Check sheet for the drawn part. Datum: minimum x, y, z corner. Units: mm. Round coordinates to 2 decimals unless told otherwise and drop trailing zeros. Write each loop counter-clockwise with the first axis right and the second up, starting at its lowest first coordinate (ties: lowest second). Pieces come first, ordered by that corner, then holes. Notation, with made-up numbers: (-11, 46) -> (41, 46) arc R17 ccw to (41, 64) -> close; hole circle Ø5 at (12.5, 40.5). An arc over 180 degrees is marked (long way). Use a Markdown table: item, result.
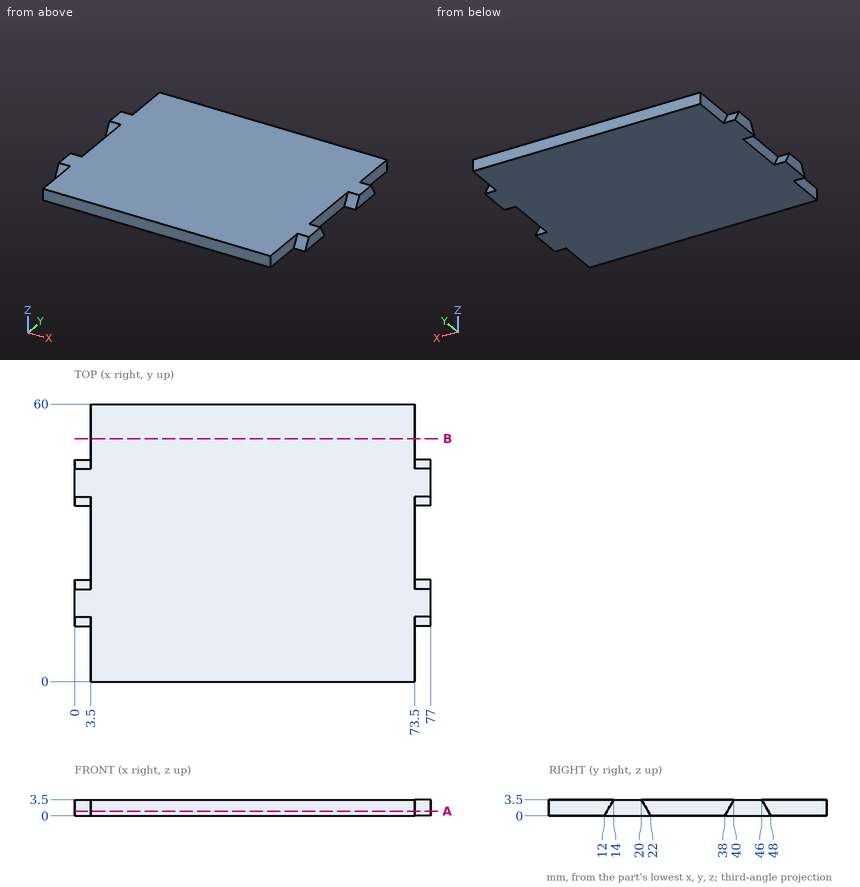
(1) Gauge pin test, flat ends, axial feed: pin 1 Ø1.8 at (y, z) = (4, 1.5) entering from +X; pin 2 Ø1.8 at (y, z) = (9.5, 2) entering from -X; pin 3 Ø2 at (x, z) = (23, 2) entering from -Y. Record the tip position at first contact, or that the pin passes through.
A:
| item | result |
|---|---|
| pin 1 | stops at x = 73.5 |
| pin 2 | stops at x = 3.5 |
| pin 3 | stops at y = 0 |
(2) Section check A-A on z = 1. Record the cut outline in (x, y).
A:
| item | result |
|---|---|
| outline | (0, 12.57) -> (3.5, 12.57) -> (3.5, 0) -> (73.5, 0) -> (73.5, 12.57) -> (77, 12.57) -> (77, 21.43) -> (73.5, 21.43) -> (73.5, 38.57) -> (77, 38.57) -> (77, 47.43) -> (73.5, 47.43) -> (73.5, 60) -> (3.5, 60) -> (3.5, 47.43) -> (0, 47.43) -> (0, 38.57) -> (3.5, 38.57) -> (3.5, 21.43) -> (0, 21.43) -> close |
(3) Thickness scan on line 1 (X direction, y = 28, z = 3). Record the ranges inside material, lowest first.
A:
| item | result |
|---|---|
| line 1 | x = 3.5 to 73.5 |
(4) Section check B-B on y = 52.5. Record the cut outline in (x, z), plus the area to 3 significant figures.
A:
| item | result |
|---|---|
| outline | (3.5, 0) -> (73.5, 0) -> (73.5, 3.5) -> (3.5, 3.5) -> close |
| area | 245 mm2 |
